```python
from build123d import *

# Parameters (mm, degrees)
SKETCH_R  = 1.5
PAD_DEPTH = 7


with BuildPart() as part:
    # Sketch → Pad (new body)
    with BuildSketch(Plane.XY):
        with BuildLine():
            Line((0, 15.997543), (24, 15.997543))
            ThreePointArc((27.998177, 11.999997), (26.8271, 14.826912), (24, 15.997543))
            ThreePointArc((27.998811, 0), (29.086586, 6.000056), (27.998177, 11.999997))
            ThreePointArc((24, -3.998177), (26.827548, -2.827362), (27.998811, 0))
            Line((0, -3.998177), (24, -3.998177))
            ThreePointArc((-3.998177, 0), (-2.827138, -2.827138), (0, -3.998177))
            ThreePointArc((-3.997546, 11.999992), (-5.086015, 6.000054), (-3.998177, 0))
            ThreePointArc((0, 15.997543), (-2.826693, 14.826687), (-3.997546, 11.999992))
        make_face()
        with Locations((-2.001505, 5.998805)):
            Circle(SKETCH_R, mode=Mode.SUBTRACT)
        with Locations((26.000681, 5.998509)):
            Circle(SKETCH_R, mode=Mode.SUBTRACT)
        Polygon((0, 0), (24.000633, 0), (24.000632, 4.5), (24.000632, 7.5), (24.000632, 11.999997), (0, 11.999997), (0, 7.5), (0, 4.5), align=None, mode=Mode.SUBTRACT)
    extrude(amount=PAD_DEPTH)


solid = part.part
```
CAD build for the part. Positions are in the model's coordinates, mm. A direction names the side the tool comes from. Coordinates: 2 decimals unless noted, no trailing zeros. Loops run counter-clockwise (first coordinate to the right, second up) from the corner with the lowest first, then second, coordinate; pieces in that order, holes last. Notation, with made-up numbers: (76.25, 80) - (90.25, 80) arc R11 ccw to (90.25, 100) - close; hole circle Ø6 at (83, 49). An arc over 180 degrees is marked (long way). Return JSON: item names as keys, results as strings.
1. Band-saw the part on A-A (x = 15). Give the cut face in (y, z), and give its area (3 significant figures).
Result:
{"outline": "(-4, 0) - (0, 0) - (0, 7) - (-4, 7) - close; (12, 0) - (16, 0) - (16, 7) - (12, 7) - close", "area": "56.0 mm2"}
2. Mould opens along X. For faces 3 (the cylindrical face through (-2.197, 7.486, 3.451)), 4 (the cylindrical face through (-5.086, 6.086, 3.451)), 5 (the flat face through (12, -1, 7)) say: released by +X, released by -X, zero draft, split by the parting line, or undercut.
Result:
{"face 3": "undercut", "face 4": "released by -X", "face 5": "zero draft"}
3. Drop flat-ended pins along their axis: pin 1 (1.3 mm diameter, centred on y = 3.5, z = 4.5, fed in from -X); pin 2 (1.5 mm diameter, centred on y = 10.5, z = 4, fed in from -X); pin 3 (2.5 mm diameter, centred on x = -2, y = 6, fed in from -Z). Give the stop position or say it passes through.
Result:
{"pin 1": "stops at x = -4.99", "pin 2": "stops at x = -4.67", "pin 3": "passes through"}
4. 3-axis set-ups, long thin cutter, end or side, ignore diameter. For faces 1 (the cylindrical face through (-2.795, 14.858, 3.451)), 2 (the flat face through (0, 6, 3)): which of +Z, -Z, +X, -X, +Y, -Y reach the whole face in a straight line?
Result:
{"face 1": "+Z, -Z, -X, +Y", "face 2": "+Z, -Z"}
5. Band-saw the part on D-D (z = 4). Give the cut face in (x, y), and give its area (3 significant figures).
Result:
{"outline": "(-4, 0) arc R4 ccw to (0, -4) - (24, -4) arc R4 ccw to (28, 0) arc R17.09 ccw to (28, 12) arc R4 ccw to (24, 16) - (0, 16) arc R4 ccw to (-4, 12) arc R17.09 ccw to start; hole circle Ø3 at (-2, 6); hole (0, 0) - (24, 0) - (24, 4.5) - (24, 12) - (0, 12) - close; hole circle Ø3 at (26, 6)", "area": "341 mm2"}
6. Band-saw the part on C-C (y = 9.75). Give the cut face in (x, z).
Result:
{"outline": "(-4.67, 0) - (0, 0) - (0, 7) - (-4.67, 7) - close; (24, 0) - (28.67, 0) - (28.67, 7) - (24, 7) - close"}
7. Probe L1, parallel to Y at x = 4.5, z = 6.5; L2, parallel to X at y = 11, z = 4.75; L3, parallel to Y at x = -1, z = 2.75. List the from-to ranges inside material, lowest first. Write a range as from..to.
Result:
{"L1": "y = -4..0, 12..16", "L2": "x = -4.34..0, 24..28.34", "L3": "y = -3.87..4.88, 7.12..15.87"}
8. Band-saw the part on B-B (y = 5.25). Give the cut face in (x, z), and give its area (3 significant figures).
Result:
{"outline": "(-5.07, 0) - (-3.3, 0) - (-3.3, 7) - (-5.07, 7) - close; (-0.7, 0) - (0, 0) - (0, 7) - (-0.7, 7) - close; (24, 0) - (24.7, 0) - (24.7, 7) - (24, 7) - close; (27.3, 0) - (29.07, 0) - (29.07, 7) - (27.3, 7) - close", "area": "34.6 mm2"}
